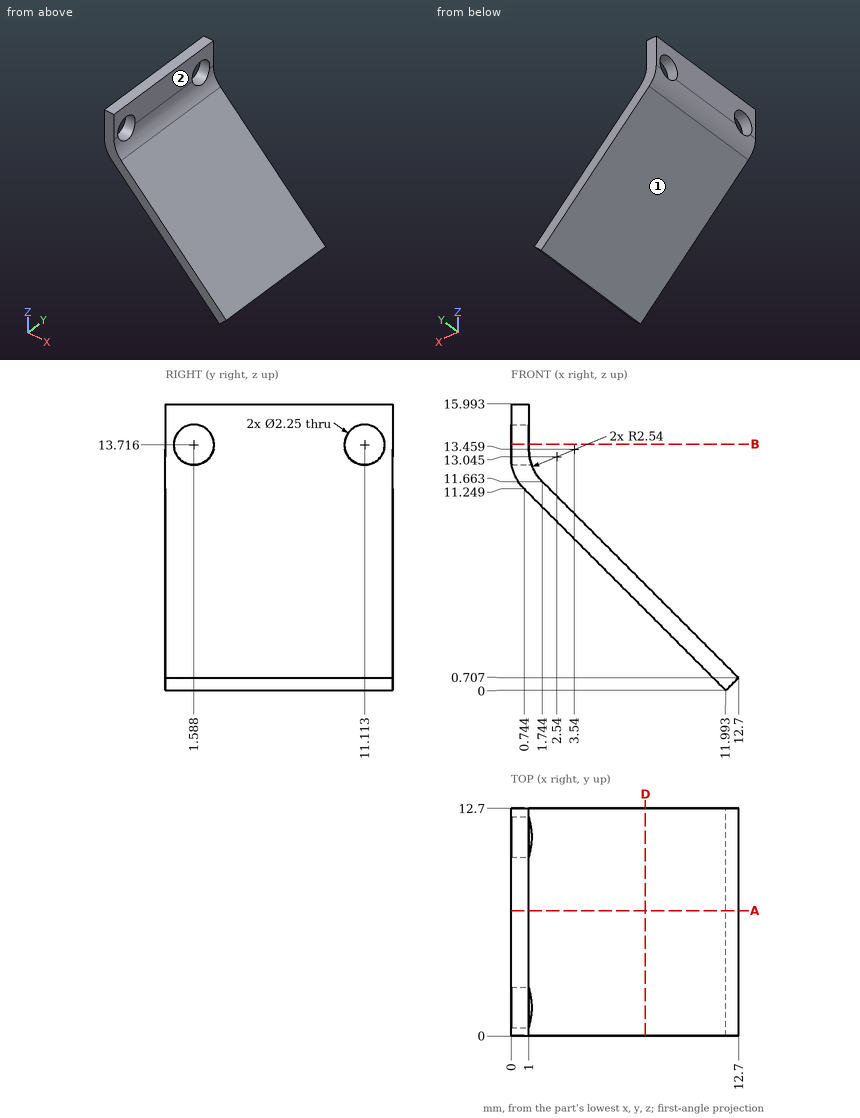
Geometry: see drawing. Coordinates: mm, zero at the bounding-box minimum. A direction names the side the tool comes from. Round coordinates to 2 decimals unless told otherwise and drop trailing zeros. Order: outer loops, then holes, each group sorted by start corner. A loop starts at its lowest first (then second) coordinate and runs counter-clockwise, first axis right, second up. Notation, with made-up numbers: (48.25, -33) -> (63.25, -33) arc R14 cw to (63.25, -17) -> close; hole circle Ø7 at (74.5, 16.25). An arc over 180 degrees is marked (long way). Use CSV: the item, a comma, the result in double quotes.
(1) Ray query, L1, parallel to X at y = 8.75, z = 15.25; L2, parallel to Z at x = 11.25, y = 11.75 (1 decimal); L3, parallel to X at y = 1.25, z = 10 (1 decimal). Return the intervals inside material, ascending.
Report:
L1,"0 to 1"
L2,"0.7 to 2.2"
L3,"2 to 3.4"
(2) Section D-D on x = 7.5. Return the cut outline in (y, z).
Report:
outline,"(0, 4.49) -> (12.7, 4.49) -> (12.7, 5.91) -> (0, 5.91) -> close"
(3) Section A-A on y = 7. Return the cut outline in (x, z) (1 decimal).
Report:
outline,"(0, 13) arc R2.5 ccw to (0.7, 11.2) -> (12, 0) -> (12.7, 0.7) -> (1.7, 11.7) arc R2.5 cw to (1, 13.5) -> (1, 16) -> (0, 16) -> close"
(4) Access query for the marked faces 1 and 2. Directions: +Z, -Z, +X, -X, +Y, -Y. A direction counts if a zero-diameter tool reaches every point of the face in a straight line with its end or side. Return the directions, or none.
Report:
face 1,"-Z, -X, +Y, -Y"
face 2,"+Z, +X, +Y, -Y"
(5) First-contact query: pin 1 Ø0.8 at (y, z) = (6, 15.5) entering from +X; pin 2 Ø3 at (y, z) = (7, 5) entering from -X; pin 3 Ø1.5 at (x, y) = (2.5, 3.5) entering from -Z; pin 4 Ø3 at (y, z) = (11.11, 13.72) entering from -X. Flat tips, straight axial feed; report the tip coordinate or a pass-through.
Report:
pin 1,"x = 1"
pin 2,"x = 5.49"
pin 3,"z = 8.74"
pin 4,"x = 0"
(6) Section B-B on z = 13.75. Return the cut outline in (x, y).
Report:
outline,"(0, 0) -> (1, 0) -> (1, 0.46) -> (0, 0.46) -> close; (0, 2.71) -> (1, 2.71) -> (1, 9.99) -> (0, 9.99) -> close; (0, 12.24) -> (1, 12.24) -> (1, 12.7) -> (0, 12.7) -> close"
